For this review, use the dimensioned drawing (mm, ordinates from the lowest corner) and the shaded views. Round coordinates to 2 decimals unless told otherwise and drop trailing zeros. Order: outer loops, then holes, each group sorted by start corner. A loop starts at its lowest first (then second) coordinate and runs counter-clockwise, first axis right, second up. Notation, with made-up numbers: (12, 2) - (53, 2) arc R34 cw to (53, 36) - close; hole circle Ø5 at (52, 7.5). An arc over 180 degrees is marked (long way). Write item = value, one per line.
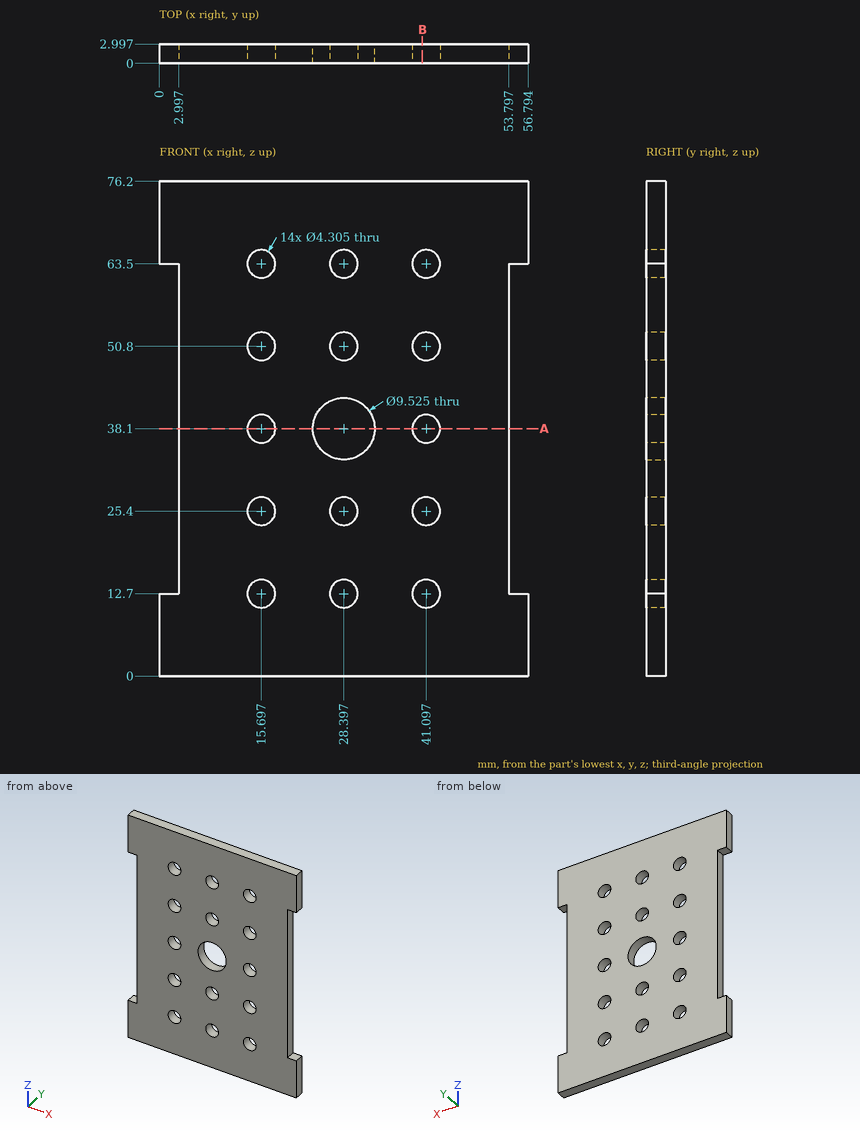
Item 1: Insertion check: P1, Ø1.5, axis at y = 2, z = 31.5, coming from the -X side; P2, Ø1.5, axis at y = 2, z = 35.5, coming from the +X side. Each pin has a flat end and moves straight along its axis. Give the tip position at first contact, or say it passes through.
Data:
P1 = 3
P2 = 53.8
Item 2: Take a section at B-B, the plane x = 40.5. State the section outline as (y, z) points.
Data:
outline = (0, 0) - (3, 0) - (3, 10.63) - (0, 10.63) - close; (0, 14.77) - (3, 14.77) - (3, 23.33) - (0, 23.33) - close; (0, 27.47) - (3, 27.47) - (3, 36.03) - (0, 36.03) - close; (0, 40.17) - (3, 40.17) - (3, 48.73) - (0, 48.73) - close; (0, 52.87) - (3, 52.87) - (3, 61.43) - (0, 61.43) - close; (0, 65.57) - (3, 65.57) - (3, 76.2) - (0, 76.2) - close
Item 3: For line 1 along X through (y, z) = (0.9, 12) (1 decimal); line 2 along Z through (x, y) = (27, 1.85) (1 decimal); line 3 along X through (y, z) = (2.15, 36.5) (1 decimal), list the stretches that pass through material, from the lowest coordinate up. Write a range as [from, to].
Data:
line_1 = [0, 13.7], [17.7, 26.4], [30.4, 39.1], [43.1, 56.8]
line_2 = [0, 11.1], [14.3, 23.8], [27, 33.5], [42.7, 49.2], [52.4, 61.9], [65.1, 76.2]
line_3 = [3, 14.3], [17.1, 23.9], [32.9, 39.7], [42.5, 53.8]
Item 4: Take a section at A-A, the plane z = 38.1. Count the separate pieces of the cut face and the enclosed holes in it.
Data:
separate_pieces = 4
enclosed_holes = 0
